For this review, use the dimensioned drawing (mm, ordinates from the lowest corner) and the shaded views. A direction names the side the tool comes from. Coordinates: 2 decimals unless noted, no trailing zeros. Order: outer loops, then holes, each group sorted by start corner. A loop starts at its lowest first (then second) coordinate and runs counter-clockwise, first axis right, second up. Notation, with made-up numbers: M 3.5,59 L 53.5,59 A23 ccw 53.5,71 Z; hole C 33.5,34.25 d11. An arc over 180 degrees is marked long. Use one line per item in the form item = value. Start each with the question number.
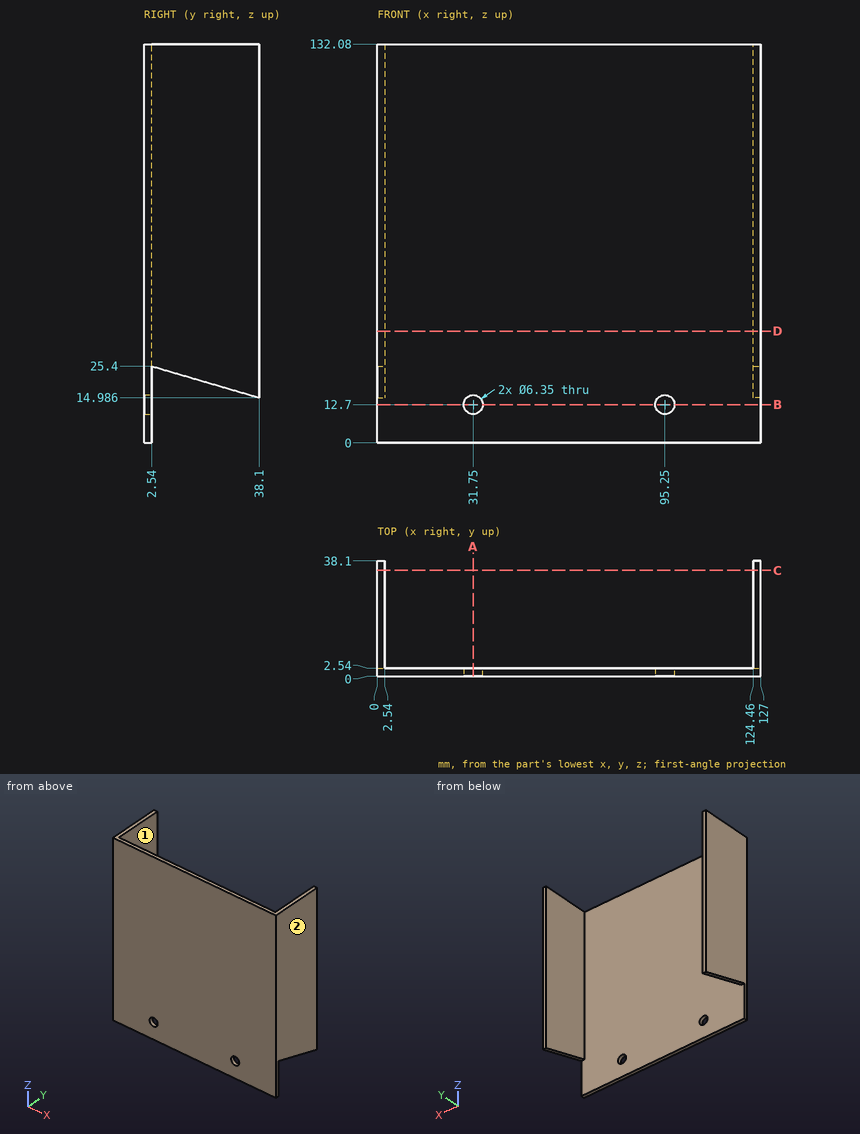
1. Consider section C-C, the plane y = 35. Write out the cut boundary in (x, z), plus the area to 3 significant figures.
2. For pin 1 Ø5 at (x, z) = (31.75, 12.7) entering from -Y; pin 2 Ø8.5 at (x, z) = (95.25, 12.7) entering from +Y, all flat-tipped, find the tip position at first contact; note any pin that passes through.
3. Tool access review of the marked faces 1 and 2: name each direction out of +Z, -Z, +X, -X, +Y, -Y from which nothing blocks a thin tool from reaching the whole face with its end or side.
4. Consider section A-A, the plane x = 31.75. Write out the cut boundary in (y, z) (3 decimals), plus the area to 3 significant figures.
5. To check wall thickness, follow line 1 (Z direction, x = 95.25, y = 1.55) (3 decimals); line 2 (X direction, y = 19, z = 92.5); line 3 (Y direction, x = 63.5, z = 126.5). State the ranges of each line that lie inside material, in increasing order.
6. Consider section D-D, the plane z = 37. Write out the cut boundary in (x, y).
7. Consider section B-B, the plane z = 12.7. Write out the cut boundary in (x, y) (3 decimals), plus the area to 3 significant figures.
Answers follow:
q1.outline = M 0,15.89 L 2.54,15.89 L 2.54,132.08 L 0,132.08 Z; M 124.46,15.89 L 127,15.89 L 127,132.08 L 124.46,132.08 Z
q1.area = 590 mm²
q2.pin_1 = through
q2.pin_2 = 2.54
q3.face_1 = +Z, -Z, +Y
q3.face_2 = +Z, -Z, +X, +Y, -Y
q4.outline = M 0,0 L 2.54,0 L 2.54,9.525 L 0,9.525 Z; M 0,15.875 L 2.54,15.875 L 2.54,132.08 L 0,132.08 Z
q4.area = 319 mm²
q5.line_1 = 0 to 9.525, 15.875 to 132.08
q5.line_2 = 0 to 2.54, 124.46 to 127
q5.line_3 = 0 to 2.54
q6.outline = M 0,0 L 127,0 L 127,38.1 L 124.46,38.1 L 124.46,2.54 L 2.54,2.54 L 2.54,38.1 L 0,38.1 Z
q7.outline = M 0,0 L 28.575,0 L 28.575,2.54 L 0,2.54 Z; M 34.925,0 L 92.075,0 L 92.075,2.54 L 34.925,2.54 Z; M 98.425,0 L 127,0 L 127,2.54 L 98.425,2.54 Z
q7.area = 290 mm²
